Verification items for the finished model (mm, model axes). A direction names the side the tool comes from. Coordinates: 2 decimals unless noted, no trailing zeros. Write each loop counter-clockwise with the first axis right and the second up, starting at its lowest first coordinate (ties: lowest second). Pieces come first, ordered by that corner, then holes. Notation, with made-up numbers: (72.25, 57) -> (77.25, 57) arc R16 ccw to (77.25, 79) -> close; hole circle Ø1 at (5, 77.5). An arc over 180 degrees is marked (long way). Answer in a Markdown table with one row per item.
Autodesk Inventor part; units mm, degrees
ref_plane "YZ Plane" through (0, 0, 0) normal (1, 0, 0) x (0, 1, 0)
ref_plane "XZ Plane" through (0, 0, 0) normal (0, 1, 0) x (-1, 0, 0)
ref_plane "XY Plane" through (0, 0, 0) normal (0, 0, 1) x (1, 0, 0)
sketch "Esquisse1" plane through (0, 0, 0) normal (0, 1, 0) x (-1, 0, 0)
  line L0 (-55, 85) -> (55, 85)
  line L1 (55, 85) -> (55, -85)
  line L2 (55, -85) -> (-55, -85)
  line L3 (-55, -85) -> (-55, 85)
  line L4 (-55, 85) -> (55, -85) construction
  line L5 (55, 85) -> (-55, -85) construction
  point P0 (0, 0)
  dimension "d0" = 170
  dimension "d1" = 110
extrude "Extrusion1" add sketch "Esquisse1" along normal blind 30
fillet "Congé1" radius 5 4 edges at (0, 30, 85) (55, 30, 0) (0, 30, -85) (-55, 30, 0)
fillet "Congé2" radius 5 8 edges at (-53.5355, 28.5355, -83.5355) (-55, 12.5, -85) (-53.5355, 28.5355, 83.5355) (-55, 12.5, 85) (53.5355, 28.5355, -83.5355) (55, 12.5, -85) (53.5355, 28.5355, 83.5355) (55, 12.5, 85)
sketch "Esquisse2" plane through (0, 30, 0) normal (0, 1, 0) x (1, 0, 0)
  line L0 (-50, -80) -> (-50, 80)
  line L1 (-50, 80) -> (50, 80)
  line L2 (-50, -80) -> (50, -80)
  line L3 (50, -80) -> (50, 80)
  line L4 (50, 80) -> (-50, 80)
  line L5 (-50, 80) -> (-50, -80)
  point P0 (0, 0)
extrude "Extrusion2" cut sketch "Esquisse2" against normal blind 25
sketch "Esquisse3" plane through (55, 0, -85) normal (0, 0, -1) x (-1, 0, 0)
  line L0 (55, 14) -> (40, 14) construction
  line L1 (105, 0) -> (0, 0) construction
  line L2 (0, 0) -> (0, 25) construction
  point P0 (55, 0)
  dimension "d15" = 14
  dimension "d16" = 15
  dimension "d17" = 40
hole "Perçage1" at (15, 14, -85) at (0, 14, -85) direction (0, 0, 1) diameter 2.459 depth 8.8 tip angle 118
sketch "Esquisse4" plane through (-50, 0, 85) normal (0, 0, 1) x (1, 0, 0)
  line L0 (45, 14) -> (60, 14) construction
  line L1 (100, 25) -> (100, 0) construction
  line L2 (100, 0) -> (0, 0) construction
  point P0 (50, 0)
  dimension "d25" = 15
  dimension "d26" = 40
  dimension "d27" = 14
hole "Perçage2" at (-5, 14, 85) at (10, 14, 85) direction (0, 0, -1) diameter 2.459 depth 8.8 tip angle 118
sketch "Esquisse5" plane through (55, 0, 80) normal (1, 0, 0) x (0, 0, -1)
  line L0 (160, 25) -> (0, 25)
  line L1 (0, 5) -> (160, 5)
  line L2 (7.5, 25) -> (27.5, 25)
  line L3 (27.5, 25) -> (27.5, 5)
  line L4 (27.5, 5) -> (7.5, 5)
  line L5 (7.5, 5) -> (7.5, 25)
  line L6 (0, 0) -> (0, 25)
  line L7 (152.5, 25) -> (132.5, 25)
  line L8 (132.5, 25) -> (132.5, 5)
  line L9 (132.5, 5) -> (152.5, 5)
  line L10 (152.5, 5) -> (152.5, 25)
  line L11 (160, 25) -> (160, 0)
  point P0 (80, 0)
  dimension "d40" = 7.5
  dimension "d41" = 20
  dimension "d42" = 7.5
  dimension "d43" = 20
extrude "Extrusion3" cut sketch "Esquisse5" against normal blind 5 contours L10 L1 L8 L0 | L3 L1 L5 L0
sketch "Esquisse6" plane through (0, 5, 0) normal (0, 1, 0) x (1, 0, 0)
  line L0 (-50, 80) -> (50, 80)
  line L1 (50, -80) -> (-50, -80)
  line L2 (25, -80) -> (30, -80)
  line L3 (50, 52.5) -> (50, -52.5)
  line L4 (50, 45) -> (10, 45)
  line L5 (10, 45) -> (10, 40)
  line L6 (10, 40) -> (50, 40)
  line L7 (50, 40) -> (50, 45)
  line L8 (10, 40) -> (5, 40)
  line L9 (5, 40) -> (5, 80)
  line L10 (5, 80) -> (10, 80)
  line L11 (10, 80) -> (10, 40)
  line L12 (55, 52.5) -> (50, 52.5)
  line L13 (50, 80) -> (50, -80)
  line L14 (10, -80) -> (5, -80)
  line L15 (5, -80) -> (5, -40)
  line L16 (5, -40) -> (10, -40)
  line L17 (10, -40) -> (10, -80)
  line L18 (50, -40) -> (10, -40)
  line L19 (10, -40) -> (10, -45)
  line L20 (10, -45) -> (50, -45)
  line L21 (50, -45) -> (50, -40)
  point P0 (0, 0)
  point P1 (7.5, -40)
  dimension "d44" = 5
  dimension "d45" = 5
  dimension "d46" = 7.5
  dimension "d47" = 40
  dimension "d48" = 5
  dimension "d49" = 7.5
  dimension "d50" = 5
  dimension "d51" = 40
extrude "Extrusion4" add sketch "Esquisse6" along normal blind 10 contours L0 L11 L5 L8 L9 | L4 L3 L6 L5 | L20 L17 L18 L3 | L1 L15 L16 L17
sketch "Esquisse8" plane through (55, 0, 80) normal (1, 0, 0) x (0, 0, -1)
  line L0 (0, 25) -> (0, 0) construction
  line L1 (0, 20) -> (3.75, 20) construction
  line L2 (3.75, 20) -> (7.5, 20) construction
  line L3 (7.5, 25) -> (7.5, 5) construction
  line L4 (3.75, 20) -> (3.75, 15) construction
  line L5 (0, 15) -> (35, 15) construction
  line L6 (3.75, 20) -> (3.75, 25) construction
  line L7 (160, 25) -> (0, 25) construction
  line L8 (31.25, 20) -> (31.25, 25) construction
  line L9 (31.25, 20) -> (27.5, 20) construction
  line L10 (27.5, 5) -> (27.5, 25) construction
  line L11 (128.75, 20) -> (128.75, 25) construction
  line L12 (128.75, 20) -> (132.5, 20) construction
  line L13 (156.25, 20) -> (156.25, 25) construction
  line L14 (156.25, 20) -> (152.5, 20) construction
  line L15 (152.5, 25) -> (152.5, 5) construction
  line L16 (132.5, 5) -> (132.5, 25) construction
  point P0 (80, 0)
hole "Perçage4" at (55, 20, 76.25) at (55, 20, 48.75) at (55, 20, -48.75) at (55, 20, -76.25) direction (-1, 0, 0) diameter 3 depth 8.8 tip angle 118
equation "\"d45\" = d44"
equation "\"d50\" = d45"
equation "\"d51\" = d47"
properties part number "P1794_001_basManette"
1. Section check B-B, the plane x = 32.5. Record the boundary of the cut face in (y, z).
Geometry says:
| item | result |
|---|---|
| outline | (0, -85) -> (25, -85) arc R5 ccw to (30, -80) -> (5, -80) -> (5, -45) -> (15, -45) -> (15, -40) -> (5, -40) -> (5, 40) -> (15, 40) -> (15, 45) -> (5, 45) -> (5, 80) -> (30, 80) arc R5 ccw to (25, 85) -> (0, 85) -> close |
2. Thickness scan on line 1 (Z direction, x = 19.5, y = 12); line 2 (Z direction, x = -21.5, y = 25.25); line 3 (X direction, y = 22, z = 19.5). Record the ranges inside material, lowest first. Write a range as from..to.
Geometry says:
| item | result |
|---|---|
| line 1 | -85..-80, -45..-40, 40..45, 80..85 |
| line 2 | -84.99..-80, 80..84.99 |
| line 3 | -55..-50, 50..55 |
3. Depth check by flat-ended pin: P1, Ø6, axis at x = -29.5, z = 61.5, coming from the +Y side; P2, Ø5, axis at y = 11, z = -54.5, coming from the +X side; P3, Ø2.5, axis at x = 51.5, y = 13, coming from the +Z side; P4, Ø3, axis at y = 9, z = 58, coming from the +X side. Enter the tip coordinate at first touch or a pass-through.
Geometry says:
| item | result |
|---|---|
| P1 | y = 5 |
| P2 | x = 55 |
| P3 | z = 84.99 |
| P4 | x = 10 |
4. Tool access check on faces 1 (the flat face through (1, 0, 1)), 2 (the flat face through (5, 10, -60)), 3 (the flat face through (53, 15, 52.5)). Record the directions out of +Z, -Z, +X, -X, +Y, -Y that give a thin tool (end or side, any length) a straight path to the whole face; none if there is none.
Geometry says:
| item | result |
|---|---|
| face 1 | +Z, -Z, +X, -X, -Y |
| face 2 | +Y |
| face 3 | +X |
5. Section check A-A, the plane z = 28. Record the boundary of the cut face in (x, y), plus the area to 3 significant figures.
Geometry says:
| item | result |
|---|---|
| outline | (-55, 0) -> (55, 0) -> (55, 25) arc R5 ccw to (50, 30) -> (50, 5) -> (-50, 5) -> (-50, 30) arc R5 ccw to (-55, 25) -> close |
| area | 789 mm^2 |
6. Mould release check, pull along X, two halves, no side actions. Record for faces 4 (the cylindrical face through (-54, 28, -1)), 5 (the flat face through (10, 10, -63)), 6 (the flat face through (53, 25, -63)): released by +X, released by -X, zero draft, split by the parting line, or undercut.
Geometry says:
| item | result |
|---|---|
| face 4 | released by -X |
| face 5 | undercut |
| face 6 | zero draft |
7. Section check D-D, the plane z = -43. Record the boundary of the cut face in (x, y).
Geometry says:
| item | result |
|---|---|
| outline | (-55, 0) -> (55, 0) -> (55, 25) arc R5 ccw to (50, 30) -> (50, 15) -> (5, 15) -> (5, 5) -> (-50, 5) -> (-50, 30) arc R5 ccw to (-55, 25) -> close |
8. Section check C-C, the plane x = -16.5. Record the boundary of the cut face in (y, z).
Geometry says:
| item | result |
|---|---|
| outline | (0, -85) -> (25, -85) arc R5 ccw to (30, -80) -> (5, -80) -> (5, 80) -> (30, 80) arc R5 ccw to (25, 85) -> (0, 85) -> close |
